```python
from build123d import *

# Parameters (mm, degrees)
BOSS_EXTRUDE1_DEPTH = 196.85


with BuildPart() as part:
    # Sketch1 → Boss-Extrude1 (new body, symmetric)
    with BuildSketch(Plane.YZ):
        with BuildLine():
            Line((-20.6375, 25.4), (20.6375, 25.4))
            ThreePointArc((20.6375, 25.4), (24.005096045, 24.005096045), (25.4, 20.6375))
            Line((25.4, 20.6375), (25.4, -20.6375))
            ThreePointArc((25.4, -20.6375), (24.005096045, -24.005096045), (20.6375, -25.4))
            Line((20.6375, -25.4), (-20.6375, -25.4))
            ThreePointArc((-20.6375, -25.4), (-24.005096045, -24.005096045), (-25.4, -20.6375))
            Line((-25.4, -20.6375), (-25.4, 20.6375))
            ThreePointArc((-25.4, 20.6375), (-24.005096045, 24.005096045), (-20.6375, 25.4))
        make_face()
        with BuildLine():
            Line((-20.6375, 22.225), (20.6375, 22.225))
            ThreePointArc((20.6375, 22.225), (21.760032015, 21.760032015), (22.225, 20.6375))
            Line((22.225, 20.6375), (22.225, -20.6375))
            ThreePointArc((22.225, -20.6375), (21.760032015, -21.760032015), (20.6375, -22.225))
            Line((20.6375, -22.225), (-20.6375, -22.225))
            ThreePointArc((-20.6375, -22.225), (-21.760032015, -21.760032015), (-22.225, -20.6375))
            Line((-22.225, -20.6375), (-22.225, 20.6375))
            ThreePointArc((-22.225, 20.6375), (-21.760032015, 21.760032015), (-20.6375, 22.225))
        make_face(mode=Mode.SUBTRACT)
    extrude(amount=BOSS_EXTRUDE1_DEPTH, both=True)


solid = part.part
```
Can you work these out from the model? Positions are in its coordinate system, mm. A direction names the side the tool comes from. Give positions to 0.01 mm unless a question says otherwise; leave off trailing zeros. Write each loop counter-clockwise with the first axis right and the second up, starting at its lowest first coordinate (ties: lowest second). Pieces come first, ordered by that corner, then holes. Notation, with made-up numbers: (17, 29.25) - (51, 29.25) arc R15 ccw to (51, 54.25) - close; hole circle Ø2 at (-9, 82.25). An arc over 180 degrees is marked (long way). Write item = value, one per line. Start each with the question number.
1. Imagine slicing it at C-C (x = 73.5). Please give me the cut outline in (y, z) (1 decimal), and give its area (3 significant figures).
2. On a 3-axis mill with a long thin cutter (end or side, diameter ignored), from which of +Z, -Z, +X, -X, +Y, -Y can I reach the whole of each face in a straight line? I mean faces 4 (the face through (3, -25.4, 0)), 5 (the face through (3, -22.225, 0)). Say none if no direction works.
3. Please list where these lines run through material, in increasing order: line 1 (Z direction, x = 61, y = 3) (3 decimals); line 2 (Z direction, x = 107.5, y = 21.5).
4. Imagine slicing it at A-A (y = 4.5). Please give me the cut outline in (x, z) (3 decimals).
5. Thinking about a two-plate mould opening in Z: for faces 1 (the face through (3, 25.4, 0)), 2 (the face through (3, 0, -25.4)), 3 (the face through (3, 0, -22.225)), which applies, released by +Z, released by -Z, zero draft, split by the parting line, or undercut?
Worked answers:
q1.outline = (-25.4, -20.6) arc R4.8 ccw to (-20.6, -25.4) - (20.6, -25.4) arc R4.8 ccw to (25.4, -20.6) - (25.4, 20.6) arc R4.8 ccw to (20.6, 25.4) - (-20.6, 25.4) arc R4.8 ccw to (-25.4, 20.6) - close; hole (-22.2, -20.6) arc R1.6 ccw to (-20.6, -22.2) - (20.6, -22.2) arc R1.6 ccw to (22.2, -20.6) - (22.2, 20.6) arc R1.6 ccw to (20.6, 22.2) - (-20.6, 22.2) arc R1.6 ccw to (-22.2, 20.6) - close
q1.area = 588 mm2
q2.face_4 = +Z, -Z, +X, -X, -Y
q2.face_5 = +X, -X
q3.line_1 = -25.4 to -22.225, 22.225 to 25.4
q3.line_2 = -25.32 to -21.97, 21.97 to 25.32
q4.outline = (-196.85, -25.4) - (196.85, -25.4) - (196.85, -22.225) - (-196.85, -22.225) - close; (-196.85, 22.225) - (196.85, 22.225) - (196.85, 25.4) - (-196.85, 25.4) - close
q5.face_1 = zero draft
q5.face_2 = released by -Z
q5.face_3 = undercut
